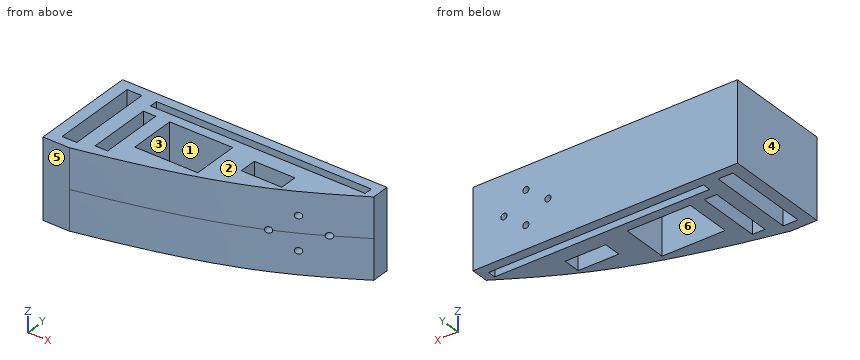
```python
from build123d import *

# Parameters (mm, degrees)
SKETCH3_W           = 8.345017316
SKETCH3_H           = 49.099302906
SKETCH3_W_2         = 121.839010914
SKETCH3_H_2         = 4.625421982
SKETCH3_W_3         = 7.122429743
SKETCH3_H_3         = 36.369854004
SKETCH3_W_4         = 35.763689771
SKETCH3_H_4         = 26.368144153
SKETCH3_W_5         = 23.034240869
SKETCH3_H_5         = 9.850168793
BOSS_EXTRUDE1_DEPTH = 22.5
CUT_EXTRUDE1_START  = -3.567987
SKETCH4_R           = 1.75
CUT_EXTRUDE1_DEPTH  = 33.567987


with BuildPart() as part:
    # Sketch3 → Boss-Extrude1 (new, symmetric)
    with BuildSketch(Plane.XY):
        with BuildLine():
            Line((0, -30), (0, 30))
            Line((0, 30), (150, 30))
            Line((150, 30), (150, 20))
            add(Edge.make_bspline(
                [(15, -30), (91.992434152, -13.820271626), (115.288714067, -0.58029396), (150, 20)],
                knots=[0, 0, 0, 0, 1, 1, 1, 1], degree=3))
            Line((15, -30), (0, -30))
        make_face()
        with Locations((10.827491342, 0.075770529)):
            Rectangle(SKETCH3_W, SKETCH3_H, mode=Mode.SUBTRACT)
        with Locations((84.244004559, 22.312710991)):
            Rectangle(SKETCH3_W_2, SKETCH3_H_2, mode=Mode.SUBTRACT)
        with Locations((26.885713974, -3.561214871)):
            Rectangle(SKETCH3_W_3, SKETCH3_H_3, mode=Mode.SUBTRACT)
        with Locations((56.208908765, 1.439640054)):
            Rectangle(SKETCH3_W_4, SKETCH3_H_4, mode=Mode.SUBTRACT)
        with Locations((100.307356745, 6.364724451)):
            Rectangle(SKETCH3_W_5, SKETCH3_H_5, mode=Mode.SUBTRACT)
    extrude(amount=BOSS_EXTRUDE1_DEPTH, both=True)

    # Sketch4 → Cut-Extrude1 (cut)
    with BuildSketch(Plane(origin=(0, 0, 0), x_dir=(1, 0, 0), z_dir=(0, 1, 0)).offset(CUT_EXTRUDE1_START)):
        with Locations(Location((107.5, 0, 0), (0, 0, 270))):
            Circle(SKETCH4_R)
        with Locations(Location((120, 9.5, 0), (0, 0, 270))):
            Circle(SKETCH4_R)
        with Locations(Location((132.5, 0, 0), (0, 0, 270))):
            Circle(SKETCH4_R)
        with Locations(Location((120, -9.5, 0), (0, 0, 270))):
            Circle(SKETCH4_R)
    extrude(amount=CUT_EXTRUDE1_DEPTH, mode=Mode.SUBTRACT)


solid = part.part
```
Check sheet for the modelled part. Datum: model origin and axes. Units: mm. Face numbers are marked on the shaded views. A direction names the side the tool comes from. Round coordinates to 2 decimals unless told otherwise and drop trailing zeros. Answer as a JSON object with one key per item and string values. Group by question number.
Q1. Gauge pin test, flat ends, axial feed: P1, Ø10, axis at x = 111, y = -6, coming from the -Z side; P2, Ø22.5, axis at x = 56.5, z = -4.5, coming from the -Y side; P3, Ø1, axis at y = -3, z = -7.5, coming from the +X side; P4, Ø2, axis at x = 120, z = 9.5, coming from the +Y side. Record the tip position at first contact, or that the pin passes through.
Q2. Mould release check, pull along X, two halves, no side actions. Record for the marked faces 1, 2, 3 and 4: released by +X, released by -X, zero draft, split by the parting line, or undercut.
Q3. Scan lines: line 1 along X through (y, z) = (26.45, 0); line 2 along X through (y, z) = (27.7, -9.5); line 3 along Y through (x, z) = (67, -17.5). Record each from-to range of solid material in increasing order. Write a range as [from, to].
Q4. Sectioned sample at A-A, the plane z = 9.5. Count the separate pieces of the cut face and the enclosed holes in it, plus the area to 3 significant figures.
Q5. Set-up check for the marked faces 5 and 6: record each of +Z, -Z, +X, -X, +Y, -Y from which the full face is reachable in a straight line by a thin tool's end or side.
Solution:
{
 "1": {"P1": "stops at z = -22.5", "P2": "stops at y = -23.13", "P3": "stops at x = 108.17", "P4": "passes through"},
 "2": {"face 1": "undercut", "face 2": "zero draft", "face 3": "undercut", "face 4": "released by -X"},
 "3": {"line 1": "x = [0, 105.75], [109.25, 130.75], [134.25, 150]", "line 2": "x = [0, 118.25], [121.75, 150]", "line 3": "y = [-17.31, -11.74], [14.62, 20], [24.63, 30]"},
 "4": {"separate pieces": "2", "enclosed holes": "4", "area": "3,800 mm²"},
 "5": {"face 5": "+Z, -Z, +X, -X, -Y", "face 6": "+Z, -Z"}
}
